Autodesk Inventor part; units mm, degrees
ref_plane "YZ Plane" through (0, 0, 0) normal (1, 0, 0) x (0, 1, 0)
ref_plane "XZ Plane" through (0, 0, 0) normal (0, 1, 0) x (-1, 0, 0)
ref_plane "XY Plane" through (0, 0, 0) normal (0, 0, 1) x (1, 0, 0)
sketch "Sketch1" plane through (0, 0, 0) normal (0, 1, 0) x (-1, 0, 0)
  line L0 (0, 0) -> (180, 0)
  line L1 (180, 0) -> (180, -220)
  line L2 (180, -220) -> (0, -220)
  line L3 (0, -220) -> (0, 0)
  line L4 (90, 0) -> (90, -220) construction
  line L5 (90, -110) -> (90, -161.5) construction
  line L6 (90, -110) -> (90, -58.5) construction
  line L7 (90, -161.5) -> (83, -161.5) construction
  line L8 (83, -161.5) -> (83, -193.1088) construction
  circle A0 centre (83, -161.5) radius 2.5
  line L9 (90, -161.5) -> (97, -161.5) construction
  circle A1 centre (97, -161.5) radius 2.5
  line L10 (90, -58.5) -> (83, -58.5) construction
  line L11 (83, -58.5) -> (83, 21.6306) construction
  circle A2 centre (83, -58.5) radius 2.5
  line L12 (90, -58.5) -> (97, -58.5) construction
  circle A3 centre (97, -58.5) radius 2.5 construction
  circle A4 centre (97, -58.5) radius 2.5
  dimension "d0" = 180
  dimension "d1" = 220
  dimension "d2" = 51.5
  dimension "d3" = 51.5
  dimension "d4" = 7
  dimension "d5" = 5
  dimension "d6" = 7
  dimension "d7" = 5
  dimension "d8" = 7
  dimension "d9" = 5
  dimension "d10" = 7
  dimension "d11" = 5
  dimension "d12" = 5
extrude "Extrusion1" add sketch "Sketch1" along normal blind 20
fillet "Fillet1" radius 20 4 edges at (0, 10, -220) (0, 10, 0) (-180, 10, -220) (-180, 10, 0)
sketch "Sketch2" plane through (0, 20, 0) normal (0, 1, 0) x (1, 0, 0)
  line L0 (-109, 173.5) -> (-71, 173.5)
  line L1 (-71, 173.5) -> (-71, 46.5)
  line L2 (-71, 46.5) -> (-109, 46.5)
  line L3 (-109, 46.5) -> (-109, 173.5)
  line L4 (0, 20) -> (0, 200)
  line L5 (-20, 220) -> (-160, 220)
  point P0 (0, 0)
  point P1 (-71, 110)
  point P2 (0, 110)
  point P3 (-90, 173.5)
  point P4 (-90, 220)
  dimension "d16" = 38
  dimension "d17" = 127
extrude "Extrusion2" cut sketch "Sketch2" against normal blind 10
fillet "Fillet2" radius 12 4 edges at (-109, 15, -173.5) (-71, 15, -173.5) (-109, 15, -46.5) (-71, 15, -46.5)
fillet "Fillet4" radius 5 8 edges at (-174.1421, 0, -214.1421) (-90, 0, -220) (-5.8579, 0, -214.1421) (0, 0, -110) (-5.8579, 0, -5.8579) (-90, 0, 0) (-174.1421, 0, -5.8579) (-180, 0, -110)
properties part number "Stand" material "Wood (Oak)"
Can you work these out from the model? Positions are in its coordinate system, mm. A direction names the side the tool comes from. Give positions to 0.01 mm unless a question says otherwise; leave off trailing zeros. Write each loop counter-clockwise with the first axis right and the second up, starting at its lowest first coordinate (ties: lowest second). Pieces come first, ordered by that corner, then holes. Notation, with made-up numbers: M -11,-27 L 38,-27 A13 ccw 38,-2 Z; hole C -35.75,-37.75 d11. An arc over 180 degrees is marked long. Answer in a Markdown table with one row per item. Add a question column.
Item 1: Imagine slicing it at B-B, the plane z = -105.5. Write out the boundary of the cut face in (x, y), plus the area to 3 significant figures.
Item 2: Please list where these lines run through material, in increasing order: L1, parallel to X at y = 5.75, z = -58.5; L2, parallel to Z at x = -97, y = 4.5; L3, parallel to Z at x = -85.5, y = 19.
Item 3: Imagine slicing it at A-A, the plane y = 14.25. Write out the boundary of the cut face in (x, z).
Item 4: On a 3-axis mill with a long thin cutter (end or side, diameter ignored), from which of +Z, -Z, +X, -X, +Y, -Y can I reach the whole of each face in a straight line? I mean faces 1 (the cylindrical face through (-80.5, 4.9, -58.6)), 2 (the flat face through (-71, 15, -111)). Say none if no direction works.
Item 5: We'd pull the mould along X, two halves only. Please class faces 3 (the cylindrical face through (-173.986, 12.605, -214.297)), 4 (the cylindrical face through (-6.014, 12.605, -5.703)), 5 (the cylindrical face through (-83, 5, -164)): released by +X, released by -X, zero draft, split by the parting line, or undercut.
Item 6: For pin 1 Ø3 at (x, y) = (-116, 8) entering from +Z; pin 2 Ø6 at (x, z) = (-83, -161.5) entering from +Y, each with a flat end and sliding along its axis, tell me the tip position at first contact or that it passes through.
Evaluation:
| question | item | result |
|---|---|---|
| 1 | outline | M -180,5 A5 ccw -175,0 L -5,0 A5 ccw 0,5 L 0,20 L -71,20 L -71,10 L -109,10 L -109,20 L -180,20 Z |
| 1 | area | 3,210 mm² |
| 2 | L1 | x = -180 to -99.5, -94.5 to -85.5, -80.5 to 0 |
| 2 | L2 | z = -219.97 to -164, -159 to -61, -56 to -0.03 |
| 2 | L3 | z = -220 to -173.5, -46.5 to 0 |
| 3 | outline | M -180,-200 A20 ccw -160,-220 L -20,-220 A20 ccw 0,-200 L 0,-20 A20 ccw -20,0 L -160,0 A20 ccw -180,-20 Z; hole M -109,-161.5 A12 ccw -97,-173.5 L -83,-173.5 A12 ccw -71,-161.5 L -71,-58.5 A12 ccw -83,-46.5 L -97,-46.5 A12 ccw -109,-58.5 Z |
| 4 | face 1 | +Y, -Y |
| 4 | face 2 | +Y |
| 5 | face 3 | released by -X |
| 5 | face 4 | released by +X |
| 5 | face 5 | undercut |
| 6 | pin 1 | stops at z = 0 |
| 6 | pin 2 | stops at y = 10 |
